from build123d import *

# Parameters (mm, degrees)
BOSS_EXTRUDE1_DEPTH = 280


with BuildPart() as part:
    # Sketch1 → Boss-Extrude1 (new body)
    with BuildSketch(Plane.XY):
        with BuildLine():
            Line((-4.5, 15), (-4.5, 14.5))
            Line((-4.5, 14.5), (-4, 14.5))
            Line((-4, 14.5), (-4, 12.8))
            Line((-4, 12.8), (-8.25, 12.8))
            Line((-8.25, 12.8), (-8.25, 9.95))
            Line((-8.25, 9.95), (-4.492893219, 6.192893219))
            ThreePointArc((-4.492893219, 6.192893219), (-4.16846987, 5.976120467), (-3.785786438, 5.9))
            Line((-3.785786438, 5.9), (3.785786438, 5.9))
            ThreePointArc((3.785786438, 5.9), (4.16846987, 5.976120467), (4.492893219, 6.192893219))
            Line((4.492893219, 6.192893219), (8.25, 9.95))
            Line((8.25, 9.95), (8.25, 12.8))
            Line((8.25, 12.8), (4, 12.8))
            Line((4, 12.8), (4, 14))
            Line((4, 14), (4.5, 14))
            Line((4.5, 14), (4.5, 15))
            Line((4.5, 15), (13, 15))
            ThreePointArc((13, 15), (14.414213562, 14.414213562), (15, 13))
            Line((15, 13), (15, 4.5))
            Line((15, 4.5), (14.5, 4.5))
            Line((14.5, 4.5), (14.5, 4))
            Line((14.5, 4), (12.8, 4))
            Line((12.8, 4), (12.8, 8.25))
            Line((12.8, 8.25), (9.95, 8.25))
            Line((9.95, 8.25), (6.192893219, 4.492893219))
            ThreePointArc((6.192893219, 4.492893219), (5.976120467, 4.16846987), (5.9, 3.785786438))
            Line((5.9, 3.785786438), (5.9, -3.785786438))
            ThreePointArc((5.9, -3.785786438), (5.976120467, -4.16846987), (6.192893219, -4.492893219))
            Line((6.192893219, -4.492893219), (9.95, -8.25))
            Line((9.95, -8.25), (12.8, -8.25))
            Line((12.8, -8.25), (12.8, -4))
            Line((12.8, -4), (14, -4))
            Line((14, -4), (14, -4.5))
            Line((14, -4.5), (15, -4.5))
            Line((15, -4.5), (15, -13))
            ThreePointArc((15, -13), (14.414213562, -14.414213562), (13, -15))
            Line((13, -15), (4.5, -15))
            Line((4.5, -15), (4.5, -14.5))
            Line((4.5, -14.5), (4, -14.5))
            Line((4, -14.5), (4, -12.8))
            Line((4, -12.8), (8.25, -12.8))
            Line((8.25, -12.8), (8.25, -9.95))
            Line((8.25, -9.95), (4.492893219, -6.192893219))
            ThreePointArc((4.492893219, -6.192893219), (4.16846987, -5.976120467), (3.785786438, -5.9))
            Line((3.785786438, -5.9), (-3.785786438, -5.9))
            ThreePointArc((-3.785786438, -5.9), (-4.16846987, -5.976120467), (-4.492893219, -6.192893219))
            Line((-4.492893219, -6.192893219), (-8.25, -9.95))
            Line((-8.25, -9.95), (-8.25, -12.8))
            Line((-8.25, -12.8), (-4, -12.8))
            Line((-4, -12.8), (-4, -14))
            Line((-4, -14), (-4.5, -14))
            Line((-4.5, -14), (-4.5, -15))
            Line((-4.5, -15), (-13, -15))
            ThreePointArc((-13, -15), (-14.414213562, -14.414213562), (-15, -13))
            Line((-15, -13), (-15, -4.5))
            Line((-15, -4.5), (-14.5, -4.5))
            Line((-14.5, -4.5), (-14.5, -4))
            Line((-14.5, -4), (-12.8, -4))
            Line((-12.8, -4), (-12.8, -8.25))
            Line((-12.8, -8.25), (-9.95, -8.25))
            Line((-9.95, -8.25), (-6.192893219, -4.492893219))
            ThreePointArc((-6.192893219, -4.492893219), (-5.976120467, -4.16846987), (-5.9, -3.785786438))
            Line((-5.9, -3.785786438), (-5.9, 3.785786438))
            ThreePointArc((-5.9, 3.785786438), (-5.976120467, 4.16846987), (-6.192893219, 4.492893219))
            Line((-6.192893219, 4.492893219), (-9.95, 8.25))
            Line((-9.95, 8.25), (-12.8, 8.25))
            Line((-12.8, 8.25), (-12.8, 4))
            Line((-12.8, 4), (-14, 4))
            Line((-14, 4), (-14, 4.5))
            Line((-14, 4.5), (-15, 4.5))
            Line((-15, 4.5), (-15, 13))
            ThreePointArc((-15, 13), (-14.414213562, 14.414213562), (-13, 15))
            Line((-13, 15), (-4.5, 15))
        make_face()
        with BuildLine():
            Line((13.3, -9.45), (9.95, -9.45))
            ThreePointArc((9.95, -9.45), (9.596446609, -9.596446609), (9.45, -9.95))
            Line((9.45, -9.95), (9.45, -13.3))
            ThreePointArc((9.45, -13.3), (9.596446609, -13.653553391), (9.95, -13.8))
            Line((9.95, -13.8), (13.3, -13.8))
            ThreePointArc((13.3, -13.8), (13.653553391, -13.653553391), (13.8, -13.3))
            Line((13.8, -13.3), (13.8, -9.95))
            ThreePointArc((13.8, -9.95), (13.653553391, -9.596446609), (13.3, -9.45))
        make_face(mode=Mode.SUBTRACT)
        with BuildLine():
            Line((9.95, 13.8), (13.3, 13.8))
            ThreePointArc((13.3, 13.8), (13.653553391, 13.653553391), (13.8, 13.3))
            Line((13.8, 13.3), (13.8, 9.95))
            ThreePointArc((13.8, 9.95), (13.653553391, 9.596446609), (13.3, 9.45))
            Line((13.3, 9.45), (9.95, 9.45))
            ThreePointArc((9.95, 9.45), (9.596446609, 9.596446609), (9.45, 9.95))
            Line((9.45, 9.95), (9.45, 13.3))
            ThreePointArc((9.45, 13.3), (9.596446609, 13.653553391), (9.95, 13.8))
        make_face(mode=Mode.SUBTRACT)
        with BuildLine():
            Line((-9.45, -13.3), (-9.45, -9.95))
            ThreePointArc((-9.45, -9.95), (-9.596446609, -9.596446609), (-9.95, -9.45))
            Line((-9.95, -9.45), (-13.3, -9.45))
            ThreePointArc((-13.3, -9.45), (-13.653553391, -9.596446609), (-13.8, -9.95))
            Line((-13.8, -9.95), (-13.8, -13.3))
            ThreePointArc((-13.8, -13.3), (-13.653553391, -13.653553391), (-13.3, -13.8))
            Line((-13.3, -13.8), (-9.95, -13.8))
            ThreePointArc((-9.95, -13.8), (-9.596446609, -13.653553391), (-9.45, -13.3))
        make_face(mode=Mode.SUBTRACT)
        with BuildLine():
            Line((-13.3, 9.45), (-9.95, 9.45))
            ThreePointArc((-9.95, 9.45), (-9.596446609, 9.596446609), (-9.45, 9.95))
            Line((-9.45, 9.95), (-9.45, 13.3))
            ThreePointArc((-9.45, 13.3), (-9.596446609, 13.653553391), (-9.95, 13.8))
            Line((-9.95, 13.8), (-13.3, 13.8))
            ThreePointArc((-13.3, 13.8), (-13.653553391, 13.653553391), (-13.8, 13.3))
            Line((-13.8, 13.3), (-13.8, 9.95))
            ThreePointArc((-13.8, 9.95), (-13.653553391, 9.596446609), (-13.3, 9.45))
        make_face(mode=Mode.SUBTRACT)
        with BuildLine():
            Line((-1.683127481, -3.2387624), (-3.111269837, -4.666904756))
            Line((-3.111269837, -4.666904756), (-4.666904756, -3.111269837))
            Line((-4.666904756, -3.111269837), (-3.2387624, -1.683127481))
            ThreePointArc((-3.2387624, -1.683127481), (-3.65, 0), (-3.2387624, 1.683127481))
            Line((-3.2387624, 1.683127481), (-4.666904756, 3.111269837))
            Line((-4.666904756, 3.111269837), (-3.111269837, 4.666904756))
            Line((-3.111269837, 4.666904756), (-1.683127481, 3.2387624))
            ThreePointArc((-1.683127481, 3.2387624), (0, 3.65), (1.683127481, 3.2387624))
            Line((1.683127481, 3.2387624), (3.111269837, 4.666904756))
            Line((3.111269837, 4.666904756), (4.666904756, 3.111269837))
            Line((4.666904756, 3.111269837), (3.2387624, 1.683127481))
            ThreePointArc((3.2387624, 1.683127481), (3.65, 0), (3.2387624, -1.683127481))
            Line((3.2387624, -1.683127481), (4.666904756, -3.111269837))
            Line((4.666904756, -3.111269837), (3.111269837, -4.666904756))
            Line((3.111269837, -4.666904756), (1.683127481, -3.2387624))
            ThreePointArc((1.683127481, -3.2387624), (0, -3.65), (-1.683127481, -3.2387624))
        make_face(mode=Mode.SUBTRACT)
    extrude(amount=BOSS_EXTRUDE1_DEPTH)


solid = part.part
Could you check a few things on this model? Use its own coordinates, in mm. A direction names the side the tool comes from. Round coordinates to 2 decimals unless told otherwise and drop trailing zeros.
Q1. Imagine slicing it at A-A, the plane z = 84. State how many separate pieces and enclosed holes the cut face has, then the cut area to 3 significant figures.
Geometry says:
separate pieces: 1
enclosed holes: 5
area: 300 mm2
Q2. I'm going to push flat-ended pins straight in: P1, Ø1.5, axis at x = 4, z = 32, coming from the -Y side; P2, Ø2, axis at y = 2, z = 233.5, coming from the +X side. Where does each tip first touch, or does it pass through?
Geometry says:
P1: stops at y = -15
P2: stops at x = 5.9
Q3. Please list where these lines run through material, in increasing order: probe 1 along Y at (x, z) = (-11.25, 250); probe 2 along Y at (x, z) = (6, 72.5).
Geometry says:
probe 1: y = -15 to -13.8, -9.45 to -8.25, 8.25 to 9.45, 13.8 to 15
probe 2: y = -15 to -12.8, -7.7 to -4.22, 4.22 to 7.7, 12.8 to 15
Q4. Thinking about a two-plate mould opening in Y: for faces 6 (the face through (-12.8, -6, 138)), 7 (the face through (0, 5.9, 138)), 8 (the face through (-15, -9, 138)), which applies, released by +Y, released by -Y, zero draft, split by the parting line, or undercut?
Geometry says:
face 6: undercut
face 7: released by +Y
face 8: zero draft
Q5. Which directions (+Z, -Z, +X, -X, +Y, -Y) give clear straight access to the entire face, cutting with the end or side of a thin tool? Please do faces 1 (the face through (9, 15, 138)), 2 (the face through (-5.9, 0, 138)), 3 (the face through (6, -12.8, 138)), 4 (the face through (5.9, 0, 138)), 5 (the face through (0, -5.9, 138)).
Geometry says:
face 1: +Z, -Z, +X, -X, +Y
face 2: +Z, -Z, -X
face 3: +Z, -Z
face 4: +Z, -Z, +X
face 5: +Z, -Z, -Y
